```python
from build123d import *

# Parameters (mm, degrees)
F0_W      = 38.1
F0_H      = 38.1
F2_DEPTH  = 38.1
F6_DEPTH  = 38.1
F8_DEPTH  = 38.1
F9_W      = 25.4
F9_H      = 7.62
F10_DEPTH = 38.1


with BuildPart() as f2:
    # F0 (on Front) → F2 (new body)
    with BuildSketch(Plane.XZ):
        with Locations((19.05, 19.05)):
            Rectangle(F0_W, F0_H)
    extrude(amount=F2_DEPTH)

    # F5 (on offset) → F6 (cut)
    with BuildSketch(Plane.YZ.offset(38.1)):
        Polygon((-6.35, 38.1), (-31.75, 38.1), (-26.67, 20.955), (-21.59, 28.575), (-16.51, 28.575), (-11.43, 20.955), align=None)
        Polygon((0, 0), (0, 38.1), (-6.35, 0), align=None)
        Polygon((-19.05, 15.875), (-25.4, 0), (-12.7, 0), align=None)
        Polygon((-31.75, 0), (-38.1, 38.1), (-38.1, 0), align=None)
    extrude(amount=-F6_DEPTH, mode=Mode.SUBTRACT)

    # F7 (on offset) → F8 (cut)
    with BuildSketch(Plane.XZ.offset(38.1)):
        Polygon((0, 38.1), (0, 0), (6.35, 38.1), align=None)
        Polygon((11.43, 16.402483), (6.35, 0), (31.75, 0), (26.67, 16.627173), (21.59, 9.525), (16.51, 9.525), align=None)
        Polygon((25.4, 38.1), (12.7, 38.1), (19.05, 22.225), align=None)
        Polygon((31.75, 38.1), (38.1, 0), (38.1, 38.1), align=None)
    extrude(amount=-F8_DEPTH, mode=Mode.SUBTRACT)

    # F9 (on offset) → F10 (cut)
    with BuildSketch(Plane.XY.offset(38.1)):
        with Locations((25.4, -11.43)):
            Rectangle(F9_W, F9_H)
        Polygon((25.4, -22.352), (0, -22.352), (0, -29.972), (1.777999, -29.972), (25.4, -29.972), align=None)
    extrude(amount=-F10_DEPTH, mode=Mode.SUBTRACT)


solid = f2.part
```
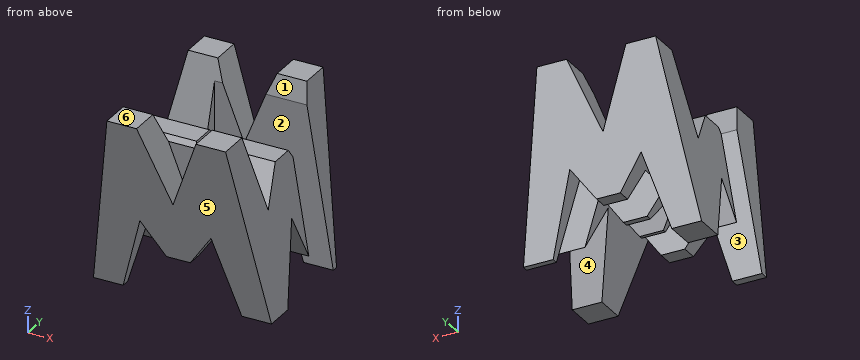
Can you work these out from the model? Positions are in its coordinate system, mm. Face numbers are marked on the shaded views. A direction names the side the tool comes from. Round coordinates to 2 decimals unless told otherwise and drop trailing zeros. Loops run counter-clockwise (first coordinate to the right, second up) from the corner with the lowest first, then second, coordinate; pieces in that order, holes last. Notation, with made-up numbers: M 75,42.25 L 118,42.25 A18 ccw 118,59.25 Z; hole C 70.25,-28 d11. An arc over 180 degrees is marked long. Write item = value, one per line. Start each with the question number.
(1) Suppose I cut it at A-A on x = 28.5. Write out the boundary of the cut face in (y, z) (3 decimals), plus the area to 3 significant figures.
(2) I'm going to push flat-ended pins straight in: P1, Ø22.5, axis at x = 20.5, z = 13, coming from the +Y side; P2, Ø4, axis at y = -27.5, z = 25, coming from the -X side; P3, Ø1, axis at x = 29, z = 11.5, coming from the -Y side; P4, Ø5, axis at y = -26, z = 34, coming from the -X side. Where does each tip first touch, or does it pass through?
(3) Suppose I cut it at C-C on x = 7.5. Write out the boundary of the cut face in (y, z) (3 decimals).
(4) I need wall thicknesses on line 1 along Y through (x, z) = (30.5, 7.5); line 2 along X through (y, z) = (-17, 11); line 3 along X through (y, z) = (-17, 13). Which ranges of each line are inside material? Lowest first, please.
(5) Which directions (+Z, -Z, +X, -X, +Y, -Y) give clear straight access to the entire face, cutting with the end or side of a thin tool? Please do the marked faces 1, 2 and 3.
(6) If we mould it in two halves opening along Y, with no side actions, what happens to the marked faces 4, 5 and 6? For each: released by +Y, released by -Y, zero draft, split by the parting line, or undercut.
Answer block:
q1.outline = M -38.1,38.1 L -33.523,10.637 L -21.145,10.637 L -19.05,15.875 L -16.955,10.637 L -15.24,10.637 L -15.24,26.67 L -16.51,28.575 L -21.59,28.575 L -26.67,20.955 L -31.75,38.1 Z; M -7.62,10.637 L -4.577,10.637 L 0,38.1 L -6.35,38.1 L -7.62,33.814 Z
q1.area = 525 mm²
q2.P1 = -2.31
q2.P2 = 25.4
q2.P3 = -33.75
q2.P4 = through
q3.outline = M -38.1,38.1 L -32.369,3.713 L -29.972,3.713 L -29.972,32.099 L -31.75,38.1 Z; M -22.352,7.62 L -19.05,15.875 L -14.185,3.713 L -5.731,3.713 L 0,38.1 L -6.35,38.1 L -11.43,20.955 L -16.51,28.575 L -21.59,28.575 L -22.352,27.432 Z
q4.line_1 = -33 to -22.4, -15.7 to -15.24, -7.62 to -5.1
q4.line_2 = 1.83 to 9.76, 15.42 to 22.65, 28.39 to 36.27
q4.line_3 = 2.17 to 10.38, 13.94 to 24.08, 27.78 to 35.93
q5.face_1 = +Z, +X, -X
q5.face_2 = +Z, -Z, +X
q5.face_3 = +Z, -Z, -X
q6.face_4 = undercut
q6.face_5 = released by -Y
q6.face_6 = zero draft
